Source: CAD feature listing. Evaluate the final solid. Frame: model axes, mm. Give positions to 0.01 mm unless a question says otherwise; leave off trailing zeros.
Autodesk Inventor part; units mm, degrees
ref_plane "YZ Plane" through (0, 0, 0) normal (1, 0, 0) x (0, 1, 0)
ref_plane "XZ Plane" through (0, 0, 0) normal (0, 1, 0) x (-1, 0, 0)
ref_plane "XY Plane" through (0, 0, 0) normal (0, 0, 1) x (1, 0, 0)
sketch "Boceto1" plane through (0, 0, 0) normal (0, 1, 0) x (-1, 0, 0)
  line L0 (100, 87.5) -> (-100, 87.5)
  line L1 (-100, 87.5) -> (-100, -87.5)
  line L2 (-100, -87.5) -> (100, -87.5)
  line L3 (100, -87.5) -> (100, 87.5)
  line L4 (100, 87.5) -> (-100, -87.5) construction
  line L5 (-100, 87.5) -> (100, -87.5) construction
  point P0 (0, 0)
  dimension "d0" = 175
  dimension "d1" = 200
extrude "Extrusión1" add sketch "Boceto1" along normal blind 3
sketch "Boceto2" plane through (0, 3, 0) normal (0, 1, 0) x (1, 0, 0)
  line L0 (-4.8, 47.5) -> (-20, 47.5)
  line L1 (-20, 47.5) -> (-20, 44.4)
  line L2 (-20, 44.4) -> (-4.8, 44.4)
  line L3 (-4.8, 44.4) -> (-4.8, 47.5)
  line L4 (100, 87.5) -> (-100, 87.5) construction
  line L5 (-100, 87.5) -> (-100, -87.5) construction
  point P0 (0, 0)
  dimension "d4" = 15.2
  dimension "d5" = 3.1
  dimension "d6" = 40
  dimension "d7" = 80
extrude "Extrusión2" cut sketch "Boceto2" against normal blind 3
fillet "Empalme1" radius 30 2 edges at (-100, 1.5, -87.5) (-100, 1.5, 87.5)
sketch "Boceto3" plane through (0, 0, 0) normal (0, -1, 0) x (1, 0, 0)
  line L0 (-70, -87.5) -> (5, -87.5)
  line L1 (5, -87.5) -> (5, -68.5)
  line L2 (5, -68.5) -> (-70, -68.5)
  line L3 (-70, -68.5) -> (-70, -87.5)
  point P0 (0, 0)
  dimension "d11" = 75
  dimension "d12" = 19
extrude "Extrusión3" cut sketch "Boceto3" against normal blind 3
mirror "Simetría1" about plane through (0, 0, 0) normal (0, 0, 1) of "Extrusión3"
fillet "Empalme3" radius 5 8 edges at (-70, 1.5, 87.5) (-70, 1.5, 68.5) (5, 1.5, 68.5) (5, 1.5, 87.5) (-70, 1.5, -87.5) (-70, 1.5, -68.5) (5, 1.5, -68.5) (5, 1.5, -87.5)
mirror "Simetría2" about plane through (0, 0, 0) normal (0, 0, 1) of "Extrusión2"
sketch "Boceto6" plane through (0, 3, 0) normal (0, 1, 0) x (1, 0, 0)
  line L0 (-100, 57.5) -> (-100, -57.5) construction
  line L1 (-10, -18.1) -> (26.2, -18.1) construction
  line L2 (-100, 0) -> (100, 0) construction
  line L3 (100, -87.5) -> (100, 87.5) construction
  line L4 (100, 87.5) -> (100, -87.5) construction
  point P0 (0, 0)
  point P1 (-10, 18.1)
  point P2 (26.2, 18.1)
  dimension "d36" = 90
  dimension "d37" = 36.2
  dimension "d38" = 36.2
  dimension "d39" = 18.1
hole "Agujero3" at (-10, 3, 18.1) at (26.2, 3, 18.1) at (-10, 3, -18.1) at (26.2, 3, -18.1) direction (0, -1, 0) diameter 4 end through all
sketch "Boceto7" plane through (0, 3, 0) normal (0, 1, 0) x (1, 0, 0)
  line L0 (-7.5, -30) -> (7.5, -30)
  line L1 (7.5, -30) -> (7.5, -25)
  line L2 (7.5, -25) -> (-7.5, -25)
  line L3 (-7.5, -25) -> (-7.5, -30)
  point P0 (0, 0)
  point P1 (0, -25)
  dimension "d47" = 5
  dimension "d48" = 15
  dimension "d49" = 25
extrude "Extrusión4" cut sketch "Boceto7" against normal blind 3
mirror "Simetría3" about plane through (0, 0, 0) normal (0, 0, 1) of "Extrusión4"
sketch "Boceto9" plane through (0, 3, 0) normal (0, 1, 0) x (1, 0, 0)
  line L0 (-85, 22.7) -> (-85, -22.7) construction
  line L1 (100, -87.5) -> (100, 87.5) construction
  line L2 (100, 0) -> (-100, 0) construction
  line L3 (-56.552, 22.7) -> (-56.552, -22.7) construction
  line L4 (-100, 57.5) -> (-100, -57.5) construction
  point P0 (0, 0)
  point P1 (-85, 0)
  dimension "d52" = 28.448
  dimension "d54" = 45.4
  dimension "d55" = 15
hole "Agujero4" at (-56.552, 3, -22.7) at (-56.552, 3, 22.7) direction (0, -1, 0) diameter 3 end through all
sketch "Boceto10" plane through (0, 3, 0) normal (0, 1, 0) x (1, 0, 0)
  line L0 (-65, -68.5) -> (0, -68.5)
  line L1 (-90, -66.5) -> (-90, 66.5) construction
  line L2 (-100, 57.5) -> (-100, -57.5) construction
  line L3 (90, -77.5) -> (15, -77.5) construction
  line L4 (90, 77.5) -> (15, 77.5) construction
  line L5 (100, -87.5) -> (100, 87.5) construction
  line L6 (5, 82.5) -> (5, 73.5) construction
  line L7 (100, 87.5) -> (10, 87.5) construction
  line L8 (10, -87.5) -> (100, -87.5) construction
  point P0 (0, 0)
  point P1 (-90, 0)
  dimension "d63" = 2
  dimension "d64" = 10
  dimension "d65" = 10
  dimension "d66" = 10
  dimension "d67" = 10
  dimension "d68" = 10
hole "Agujero5" at (90, 3, -77.5) at (15, 3, -77.5) at (90, 3, 77.5) at (15, 3, 77.5) at (-90, 3, -66.5) at (-90, 3, 66.5) direction (0, -1, 0) diameter 3 end through all
properties part number "Base_Carro"
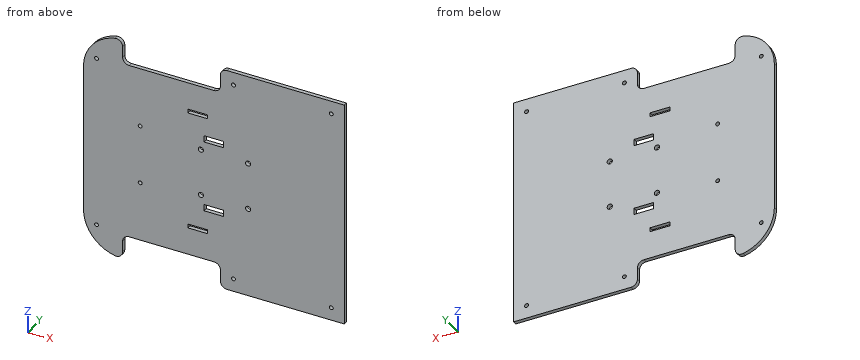
1) Cut plane A-A (y = 2.25). State how many separate pieces and enclosed holes the cut face has, and give its area (3 significant figures).
Checks:
separate pieces: 1
enclosed holes: 16
area: 31,400 mm2
2) Contact query for flat-ended pins moving along their axis: P1, Ø0.9, axis at x = -34.5, y = 1.5, coming from the -Z side; P2, Ø0.9, axis at x = -32.5, y = 1.5, coming from the +Z side; P3, Ø0.9, axis at y = 1, z = 76.5, coming from the -X side. Output: stop coordinate, or through.
Checks:
P1: stops at z = -68.5
P2: stops at z = 68.5
P3: stops at x = -93.58
3) Ray query, probe 1 along Z at (x, y) = (90, 0.7); probe 2 along X at (y, z) = (1.55, -77.5); probe 3 along X at (y, z) = (1.15, 26.5). Return the intervals inside material, ascending.
Checks:
probe 1: z = -87.5 to -79, -76 to 76, 79 to 87.5
probe 2: x = -92.36 to -70, 5 to 13.5, 16.5 to 88.5, 91.5 to 100
probe 3: x = -100 to -7.5, 7.5 to 100
